CAD build for the part. Positions are in the model's coordinates, mm. A direction names the side the tool comes from. Give positions to 0.01 mm unless a question says otherwise; leave off trailing zeros. Write each loop counter-clockwise with the first axis right and the second up, starting at its lowest first coordinate (ties: lowest second). Pieces come first, ordered by that corner, then holes. Notation, with made-up numbers: M 15.5,57 L 40.5,57 A37 ccw 40.5,95 Z; hole C -3,2.5 d9. An arc over 180 degrees is marked long. One line per question, with ' | ' between items. Start each with the question number.
1. Cut at B-B, the plane y = 10. Write the cut outline in (x, z), then the cut area to 3 significant figures.
2. Flat gauge pins, fed straight in: pin 1 (1.5 mm diameter, centred on x = -5, z = 16.5, fed in from -Y); pin 2 (2 mm diameter, centred on x = -8, z = 9, fed in from -Y); pin 3 (7.5 mm diameter, centred on y = 15, z = 11, fed in from -X); pin 4 (12 mm diameter, centred on x = -2, y = 27.5, fed in from +Z). Where does each tip first touch, or does it go through?
3. Which spindle directions (+Z, -Z, +X, -X, +Y, -Y) get a long thin tool onto all of the face, cutting with end or side? Do faces 1 (the face through (13.436, 29, 16)), 2 (the face through (12.7, 13, 13)), 3 (the face through (-6.08, 30.23, 12.88)). Say none if no direction does.
4. Cut at A-A, the plane z = 11. Write the cut outline in (x, y) (3 decimals), then the cut area to 3 significant figures.
5. Wall check: L1, parallel to X at y = 14, z = 11; L2, parallel to X at y = 27, z = 21.5; L3, parallel to Y at x = 19.5, z = 18.75. Give the ranges that are in metal, low to high.
6. Cut at C-C, the plane x = 21. Write the cut outline in (y, z) (3 decimals).
```python
from build123d import *

# Parameters (mm, degrees)
F1_DEPTH = 25.4
F3_DEPTH = 11.938
F5_DEPTH = 12.7


with BuildPart() as f1:
    # F0 (on Top) → F1 (new body)
    with BuildSketch(Plane.XY):
        Polygon((0, 25.4), (0, 0), (12.699998, 0), (12.699998, 25.4), (26.136232, 25.4), (26.136232, 44.45), (-11.963768, 44.45), (-11.963768, 25.4), align=None)
    extrude(amount=F1_DEPTH)

    # F2 (on face) → F3 (cut)
    with BuildSketch(Plane(origin=(-11.963768, 0, 0), x_dir=(0, -1, 0), z_dir=(-1, 0, 0))):
        Polygon((-34.925, 25.4), (-25.4, 0), (-25.4, 25.4), align=None)
    extrude(amount=-F3_DEPTH, mode=Mode.SUBTRACT)

    # F4 (on face) → F5 (cut)
    with BuildSketch(Plane.YZ.offset(26.136232)):
        Polygon((25.4, 25.4), (25.4, 0), (34.925, 25.4), align=None)
    extrude(amount=-F5_DEPTH, mode=Mode.SUBTRACT)


solid = f1.part
```
Here are the results:
1) outline: M 0,0 L 12.7,0 L 12.7,25.4 L 0,25.4 Z | area: 323 mm^2
2) pin 1: y = 31.31 | pin 2: y = 28.4 | pin 3: x = 0 | pin 4: z = 25.4
3) face 1: +Z, +X, -Y | face 2: +Z, -Z, +X, -Y | face 3: +Z, -X, -Y
4) outline: M -11.964,29.525 L -0.026,29.525 L -0.026,25.4 L 0,25.4 L 0,0 L 12.7,0 L 12.7,25.4 L 13.436,25.4 L 13.436,29.525 L 26.136,29.525 L 26.136,44.45 L -11.964,44.45 Z | area: 947 mm^2
5) L1: 0 to 12.7 | L2: -0.03 to 13.44 | L3: 32.43 to 44.45
6) outline: M 25.4,0 L 44.45,0 L 44.45,25.4 L 34.925,25.4 Z
